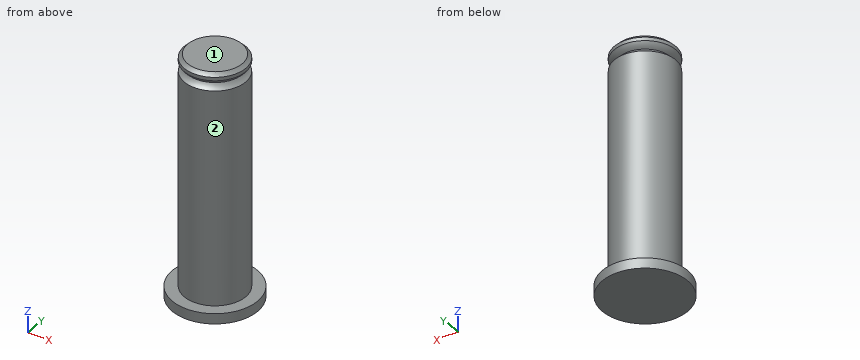
Autodesk Inventor part; units mm, degrees
ref_plane "YZ Plane" through (0, 0, 0) normal (1, 0, 0) x (0, 1, 0)
ref_plane "XZ Plane" through (0, 0, 0) normal (0, 1, 0) x (-1, 0, 0)
ref_plane "XY Plane" through (0, 0, 0) normal (0, 0, 1) x (1, 0, 0)
sketch "Sketch1" plane through (0, 0, 0) normal (0, 0, 1) x (1, 0, 0)
  circle A0 centre (0, 0) radius 6.25
  dimension "d0" = 12.5
extrude "Extrusion1" add sketch "Sketch1" along normal blind 1.5
sketch "Sketch2" plane through (0, 0, 1.5) normal (0, 0, 1) x (1, 0, 0)
  circle A0 centre (0, 0) radius 6.25
  circle A1 centre (0, 0) radius 4.5
  dimension "d3" = 9
extrude "Extrusion2" add sketch "Sketch2" along normal blind 31.4 contours A1
sketch "Sketch3" plane through (0, 0, 32.9) normal (0, 0, 1) x (1, 0, 0)
  circle A0 centre (0, 0) radius 4.5
  circle A1 centre (0, 0) radius 3.75
  dimension "d6" = 7.5
extrude "Extrusion3" add sketch "Sketch3" along normal blind 0.75 contours A1
fillet "Fillet1" radius 2 1 edges at (-3.75, 0, 32.9)
sketch "Sketch4" plane through (0, 0, 33.65) normal (0, 0, 1) x (1, 0, 0)
  circle A0 centre (0, 0) radius 4.5
  dimension "d10" = 9
extrude "Extrusion4" add sketch "Sketch4" along normal blind 0.75
fillet "Fillet2" radius 2 1 edges at (-4.5, 0, 33.65)
sketch "Sketch5" plane through (0, 0, 34.4) normal (0, 0, 1) x (1, 0, 0)
  circle A0 centre (0, 0) radius 4.5
  dimension "d14" = 9
extrude "Extrusion5" add sketch "Sketch5" along normal blind 0.5
sketch "Sketch6" plane through (0, 0, 34.9) normal (0, 0, 1) x (1, 0, 0)
  circle A0 centre (0, 0) radius 4
  dimension "d17" = 8
extrude "Extrusion6" add sketch "Sketch6" along normal blind 0.5
fillet "Fillet3" radius 3 1 edges at (-4, 0, 34.9)
properties part number "Long Pin_3DPrint"
The model under review builds one solid part; all positions refer to its coordinate system, in mm. Face numbers are marked on the shaded views. A direction names the side the tool comes from. Round coordinates to 2 decimals unless told otherwise and drop trailing zeros. Write each loop counter-clockwise with the first axis right and the second up, starting at its lowest first coordinate (ties: lowest second). Pieces come first, ordered by that corner, then holes. Notation, with made-up numbers: M 82,-21.75 L 99,-21.75 A23 cw 99,3.25 Z; hole C 81.25,77 d1. An arc over 180 degrees is marked long. Use a Markdown table: item, result. Add a question column.
Q1. We need section D-D, the plane y = 5.75. State the section outline as (x, z) points, plus the area to 3 significant figures.
Q2. Insertion check: pin 1 (5 mm diameter, centred on y = 4.5, z = 24.5, fed in from +X); pin 2 (2 mm diameter, centred on x = 1, z = 9.5, fed in from -Y); pin 3 (3 mm diameter, centred on y = 2, z = 17.5, fed in from -X). Each pin has a flat end and moves straight along its axis. Give the tip position at first contact, or say it passes through.
Q3. We need section A-A, the plane x = 0. State the section outline as (y, z) points.
Q4. To check wall thickness, follow line 1 (X direction, y = -0.25, z = 2.5); line 2 (Z direction, x = 2.5, y = -4); line 3 (Z direction, x = -3.5, y = -2.5). State the ranges of each line that lie inside material, in increasing order.
Q5. We need section C-C, the plane z = 26.5. State the section outline as (x, y) points, plus the area to 3 significant figures.
Q6. Machinability: for the marked faces 1 and 2, which of the approach directions +Z, -Z, +X, -X, +Y, -Y give a long, thin tool a straight path to every point of the face, cutting with its end or side? Answer none if there is none.
Findings below:
| question | item | result |
|---|---|---|
| 1 | outline | M -2.45,0 L 2.45,0 L 2.45,1.5 L -2.45,1.5 Z |
| 1 | area | 7.35 mm² |
| 2 | pin 1 | stops at x = 4.03 |
| 2 | pin 2 | stops at y = -4.5 |
| 2 | pin 3 | stops at x = -4.47 |
| 3 | outline | M -6.25,0 L 6.25,0 L 6.25,1.5 L 4.5,1.5 L 4.5,32.9 A2 cw 3.75,33.65 A2 ccw 4.5,34.4 L 4.5,34.9 A3 cw 4,35.4 L -4,35.4 A3 cw -4.5,34.9 L -4.5,34.4 A2 ccw -3.75,33.65 A2 cw -4.5,32.9 L -4.5,1.5 L -6.25,1.5 Z |
| 4 | line 1 | x = -4.49 to 4.49 |
| 4 | line 2 | z = 0 to 1.5 |
| 4 | line 3 | z = 0 to 33.03, 34.11 to 35.07 |
| 5 | outline | C 0,0 d9 |
| 5 | area | 63.6 mm² |
| 6 | face 1 | +Z, +X, -X, +Y, -Y |
| 6 | face 2 | +Z |
